CAD build for the part. Positions are in the model's coordinates, mm. Face numbers are marked on the shaded views. A direction names the side the tool comes from. Give positions to 0.01 mm unless a question says otherwise; leave off trailing zeros. Order: outer loops, then holes, each group sorted by start corner. A loop starts at its lowest first (then second) coordinate and runs counter-clockwise, first axis right, second up.
Item 1: Wall check: L1, parallel to X at y = 39, z = 24; L2, parallel to X at y = 15, z = 13.25; L3, parallel to Y at x = -19.5, z = 21.5. Give the ranges that are in metal, low to high.
Item 2: Band-saw the part on B-B on z = 4.75. Give the cut face in (x, y).
Item 3: Band-saw the part on A-A on z = 20.5. Give the cut face in (x, y).
Item 4: Two-plate mould, pull along Y, no slides. Class the marked faces 1, 2 and 3: released by +Y, released by -Y, zero draft, split by the parting line, or undercut.
Item 5: Which spindle directions (+Z, -Z, +X, -X, +Y, -Y) get a long thin tool onto all of the face, cutting with end or side? Do the marked faces 4, 5 and 6. Say none if no direction does.
Item 6: Band-saw the part on C-C on x = 11. Give the cut face in (y, z).
Item 7: Band-saw the part on D-D on y = 7. Give the cut face in (x, z).
Item 8: Flat gauge pins, fed straight in: P1, Ø7.5, axis at y = 57.5, z = 13.5, coming from the +X side; P2, Ø15.5, axis at x = -12, y = 21, coming from the +Z side; P3, Ø0.9, axis at x = 1.5, z = 9, coming from the +Y side. Where does each tip first touch, or does it go through?
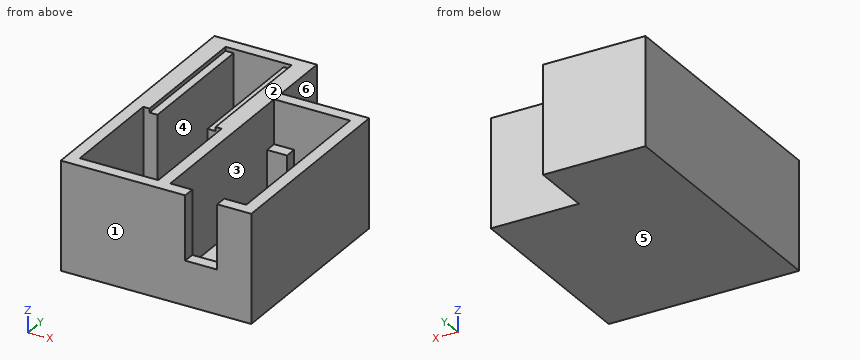
```python
from build123d import *

# Parameters (mm, degrees)
SKETCH1_W           = 2
SKETCH1_H           = 32.4
SKETCH1_W_2         = 5
SKETCH1_H_2         = 3
SKETCH1_W_3         = 3
SKETCH1_W_4         = 8
BOSS_EXTRUDE1_DEPTH = 3
BOSS_EXTRUDE2_DEPTH = 27
SKETCH1_4_W         = 5
SKETCH1_4_H         = 3
SKETCH1_4_W_2       = 3
BOSS_EXTRUDE3_DEPTH = 16
SKETCH1_5_W         = 8
SKETCH1_5_H         = 3
BOSS_EXTRUDE4_DEPTH = 11
SKETCH1_6_W         = 2
SKETCH1_6_H         = 32.4
BOSS_EXTRUDE5_DEPTH = 26


with BuildPart() as part:
    # Sketch1 → Boss-Extrude1 (new body)
    with BuildSketch(Plane.XY):
        Polygon((3, 0), (0, 0), (-3, 0), (-22.6, 0), (-22.6, 27), (-25.6, 27), (-25.6, -3), (0, -3), (5.5, -3), (5.5, 0), align=None)
        Polygon((0, 62.4), (0, 47.2), (0, 44.2), (0, 41.2), (0, 3), (0, 0), (-3, 0), (-3, 27), (-4.55, 27), (-4.55, 59.4), (-21.05, 59.4), (-21.05, 27), (-22.6, 27), (-25.6, 27), (-25.6, 59.4), (-25.6, 62.4), (-4.55, 62.4), align=None)
        with Locations((-20.05, 43.2)):
            Rectangle(SKETCH1_W, SKETCH1_H)
        Polygon((-22.6, 0), (-3, 0), (-3, 27), (-4.55, 27), (-6.55, 27), (-6.55, 59.4), (-19.05, 59.4), (-19.05, 27), (-21.05, 27), (-22.6, 27), align=None)
        with Locations((2.5, 42.7)):
            Rectangle(SKETCH1_W_2, SKETCH1_H_2)
        Polygon((0, 47.2), (0, 44.2), (5, 44.2), (14, 44.2), (19, 44.2), (19, 41.2), (19, 3), (19, 0), (22, 0), (22, 44.2), (22, 47.2), align=None)
        with Locations((16.5, 42.7)):
            Rectangle(SKETCH1_W_2, SKETCH1_H_2)
        Polygon((3, 3), (3, 0), (5.5, 0), (13.5, 0), (16, 0), (16, 3), (19, 3), (19, 41.2), (14, 41.2), (14, 44.2), (5, 44.2), (5, 41.2), (0, 41.2), (0, 3), align=None)
        with Locations((17.5, 1.5)):
            Rectangle(SKETCH1_W_3, SKETCH1_H_2)
        Polygon((16, 0), (13.5, 0), (13.5, -3), (22, -3), (22, 0), (19, 0), align=None)
        with Locations((1.5, 1.5)):
            Rectangle(SKETCH1_W_3, SKETCH1_H_2)
        with Locations((9.5, -1.5)):
            Rectangle(SKETCH1_W_4, SKETCH1_H_2)
        with Locations((-5.55, 43.2)):
            Rectangle(SKETCH1_W, SKETCH1_H)
    extrude(amount=BOSS_EXTRUDE1_DEPTH)

    # Sketch1_3 → Boss-Extrude2 (add)
    with BuildSketch(Plane.XY):
        Polygon((0, 62.4), (0, 47.2), (0, 44.2), (0, 41.2), (0, 3), (0, 0), (-3, 0), (-3, 27), (-4.55, 27), (-4.55, 59.4), (-21.05, 59.4), (-21.05, 27), (-22.6, 27), (-25.6, 27), (-25.6, 59.4), (-25.6, 62.4), (-4.55, 62.4), align=None)
        Polygon((3, 0), (0, 0), (-3, 0), (-22.6, 0), (-22.6, 27), (-25.6, 27), (-25.6, -3), (0, -3), (5.5, -3), (5.5, 0), align=None)
        Polygon((16, 0), (13.5, 0), (13.5, -3), (22, -3), (22, 0), (19, 0), align=None)
        Polygon((0, 47.2), (0, 44.2), (5, 44.2), (14, 44.2), (19, 44.2), (19, 41.2), (19, 3), (19, 0), (22, 0), (22, 44.2), (22, 47.2), align=None)
    extrude(amount=BOSS_EXTRUDE2_DEPTH)

    # Sketch1_4 → Boss-Extrude3 (add)
    with BuildSketch(Plane.XY):
        with Locations((2.5, 42.7)):
            Rectangle(SKETCH1_4_W, SKETCH1_4_H)
        with Locations((16.5, 42.7)):
            Rectangle(SKETCH1_4_W, SKETCH1_4_H)
        with Locations((17.5, 1.5)):
            Rectangle(SKETCH1_4_W_2, SKETCH1_4_H)
        with Locations((1.5, 1.5)):
            Rectangle(SKETCH1_4_W_2, SKETCH1_4_H)
    extrude(amount=BOSS_EXTRUDE3_DEPTH)

    # Sketch1_5 → Boss-Extrude4 (add)
    with BuildSketch(Plane.XY):
        with Locations((9.5, -1.5)):
            Rectangle(SKETCH1_5_W, SKETCH1_5_H)
    extrude(amount=BOSS_EXTRUDE4_DEPTH)

    # Sketch1_6 → Boss-Extrude5 (add)
    with BuildSketch(Plane.XY):
        with Locations((-5.55, 43.2)):
            Rectangle(SKETCH1_6_W, SKETCH1_6_H)
        with Locations((-20.05, 43.2)):
            Rectangle(SKETCH1_6_W, SKETCH1_6_H)
    extrude(amount=BOSS_EXTRUDE5_DEPTH)


solid = part.part
```
The answers:
1. L1: x = -25.6 to -19.05, -6.55 to 0, 19 to 22
1. L2: x = -25.6 to -22.6, -3 to 0, 19 to 22
1. L3: y = -3 to 0, 27 to 62.4
2. outline: (-25.6, -3) - (22, -3) - (22, 47.2) - (0, 47.2) - (0, 62.4) - (-25.6, 62.4) - close; hole (-22.6, 0) - (-3, 0) - (-3, 27) - (-6.55, 27) - (-6.55, 59.4) - (-19.05, 59.4) - (-19.05, 27) - (-22.6, 27) - close; hole (0, 3) - (3, 3) - (3, 0) - (16, 0) - (16, 3) - (19, 3) - (19, 41.2) - (14, 41.2) - (14, 44.2) - (5, 44.2) - (5, 41.2) - (0, 41.2) - close
3. outline: (-25.6, -3) - (5.5, -3) - (5.5, 0) - (0, 0) - (0, 44.2) - (19, 44.2) - (19, 0) - (13.5, 0) - (13.5, -3) - (22, -3) - (22, 47.2) - (0, 47.2) - (0, 62.4) - (-25.6, 62.4) - close; hole (-22.6, 0) - (-3, 0) - (-3, 27) - (-6.55, 27) - (-6.55, 59.4) - (-19.05, 59.4) - (-19.05, 27) - (-22.6, 27) - close
4. face 1: released by -Y
4. face 2: zero draft
4. face 3: undercut
5. face 4: +Z
5. face 5: -Z, +X, -X, +Y, -Y
5. face 6: +Z, -Z, +X, +Y
6. outline: (-3, 0) - (47.2, 0) - (47.2, 27) - (44.2, 27) - (44.2, 3) - (0, 3) - (0, 11) - (-3, 11) - close
7. outline: (-25.6, 0) - (22, 0) - (22, 27) - (19, 27) - (19, 3) - (0, 3) - (0, 27) - (-3, 27) - (-3, 3) - (-22.6, 3) - (-22.6, 27) - (-25.6, 27) - close
8. P1: stops at x = 0
8. P2: stops at z = 3
8. P3: stops at y = 47.2
